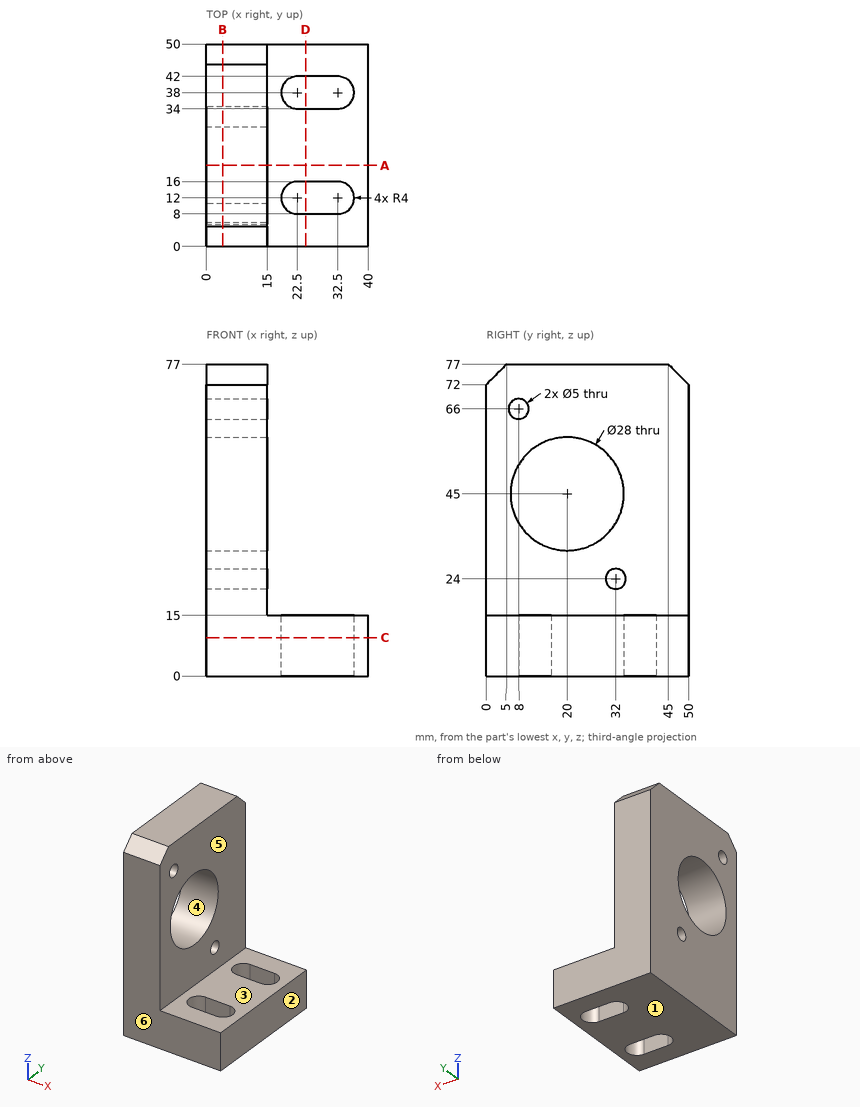
Study the drawing (mm; zero at the part's minimum x, y, z) and answer. A direction names the side the tool comes from. Coordinates: 2 decimals unless noted, no trailing zeros. Loops run counter-clockwise (first coordinate to the right, second up) from the corner with the lowest first, then second, coordinate; pieces in that order, holes last. Notation, with made-up numbers: M -30.5,-32 L -26.5,-32 A8 cw -26.5,-28 Z; hole C 33.5,80 d8. An arc over 180 degrees is marked long. Answer in a Markdown table with one row per item. Add a question column.
1. Find section B-B, the plane x = 4. Write down the section's boundary in (y, z).
2. A tool of negligible diameter and unlimited length cuts with its end or side. For the marked faces 5 and 6, from which of +Z, -Z, +X, -X, +Y, -Y can it reach the whole face along a straight path? Write none if from no direction.
3. Find section C-C, the plane z = 9.5. Write down the section's boundary in (x, y), then the cut area to 3 significant figures.
4. Find section A-A, the plane y = 20. Write down the section's boundary in (x, z).
5. Consider L1, parallel to Z at x = 14.5, y = 19.5; L2, parallel to Z at x = 7, y = 8; L3, parallel to Z at x = 10, y = 32. Determine where each line is inside the solid, lowest interval first.
6. Find section D-D, the plane x = 24.5. Write down the section's boundary in (y, z), then the cut area to 3 significant figures.
7. The mould has two halves that part along Z. Classify the marked faces 1, 2, 3 and 4: pulls with the +Z half, pulls with the -Z half, needs draft (parallel to the pull), parting line crosses it, or undercut.
8. Flat-ended cylindrical pins translate along their axes: P1, Ø25, axis at y = 20.5, z = 49.5, coming from the +X side; P2, Ø7.5, axis at x = 26, y = 20.5, coming from the +Z side. Find the tip coordinate at first contact, or state that the pin passes through.
Reported:
| question | item | result |
|---|---|---|
| 1 | outline | M 0,0 L 50,0 L 50,72 L 45,77 L 5,77 L 0,72 Z; hole C 8,66 d5; hole C 20,45 d28; hole C 32,24 d5 |
| 2 | face 5 | +Z, +X, +Y, -Y |
| 2 | face 6 | +Z, -Z, +X, -X, -Y |
| 3 | outline | M 0,0 L 40,0 L 40,50 L 0,50 Z; hole M 22.5,8 L 32.5,8 A4 ccw 32.5,16 L 22.5,16 A4 ccw Z; hole M 22.5,34 L 32.5,34 A4 ccw 32.5,42 L 22.5,42 A4 ccw Z |
| 3 | area | 1,740 mm^2 |
| 4 | outline | M 0,0 L 40,0 L 40,15 L 15,15 L 15,31 L 0,31 Z; M 0,59 L 15,59 L 15,77 L 0,77 Z |
| 5 | L1 | z = 0 to 31.01, 58.99 to 77 |
| 5 | L2 | z = 0 to 37.79, 52.21 to 63.5, 68.5 to 77 |
| 5 | L3 | z = 0 to 21.5, 26.5 to 37.79, 52.21 to 77 |
| 6 | outline | M 0,0 L 8,0 L 8,15 L 0,15 Z; M 16,0 L 34,0 L 34,15 L 16,15 Z; M 42,0 L 50,0 L 50,15 L 42,15 Z |
| 6 | area | 510 mm^2 |
| 7 | face 1 | pulls with the -Z half |
| 7 | face 2 | needs draft |
| 7 | face 3 | pulls with the +Z half |
| 7 | face 4 | undercut |
| 8 | P1 | stops at x = 15 |
| 8 | P2 | stops at z = 15 |
